The model under review builds one solid part; all positions refer to its coordinate system, in mm. A direction names the side the tool comes from. Coordinates: 2 decimals unless noted, no trailing zeros. Order: outer loops, then holes, each group sorted by start corner. A loop starts at its lowest first (then second) coordinate and runs counter-clockwise, first axis right, second up. Notation, with made-up numbers: M 78,89 L 124,89 A22 ccw 124,100 Z; hole C 74.25,-17.5 d11. An arc over 180 degrees is marked long. Answer in a Markdown table with one row per item.
from build123d import *

# Parameters (mm, degrees)
F0_W     = 66
F0_H     = 50
F1_DEPTH = 50
F2_W     = 24
F2_H     = 15
F3_DEPTH = 66
F6_DEPTH = 66
F7_W     = 16
F7_H     = 16
F8_DEPTH = 50


with BuildPart() as f1:
    # F0 (on Top) → F1 (new body)
    with BuildSketch(Plane.XY):
        with Locations((-18.661186, 12.861842)):
            Rectangle(F0_W, F0_H)
    extrude(amount=F1_DEPTH)

    # F2 (on face) → F3 (cut)
    with BuildSketch(Plane.YZ.offset(14.338814)):
        with Locations((12.148024, 42.5)):
            Rectangle(F2_W, F2_H)
    extrude(amount=-F3_DEPTH, mode=Mode.SUBTRACT)

    # F5 (on face) → F6 (cut)
    with BuildSketch(Plane.YZ.offset(14.338814)):
        with BuildLine():
            ThreePointArc((12.861842, 10.881519), (16.922608, 12.732394), (18.582238, 16.875001))
            ThreePointArc((18.582238, 16.875001), (8.241868, 21.017607), (12.861842, 10.881519))
        make_face()
    extrude(amount=-F6_DEPTH, mode=Mode.SUBTRACT)

    # F7 (on face) → F8 (cut)
    with BuildSketch(Plane.XY.offset(35)):
        with Locations((-33.807651, 12.345139)):
            Rectangle(F7_W, F7_H)
        with Locations((-3.504306, 12.252815)):
            Rectangle(F7_W, F7_H)
    extrude(amount=-F8_DEPTH, mode=Mode.SUBTRACT)


solid = f1.part
(1) Take a section at D-D (z = 27.5). Write out the cut boundary in (x, y).
Report:
| item | result |
|---|---|
| outline | M -51.66,-12.14 L 14.34,-12.14 L 14.34,37.86 L -51.66,37.86 Z; hole M -41.81,4.35 L -25.81,4.35 L -25.81,20.35 L -41.81,20.35 Z; hole M -11.5,4.25 L 4.5,4.25 L 4.5,20.25 L -11.5,20.25 Z |
(2) To check wall thickness, follow line 1 (X direction, y = 8, z = 7); line 2 (Y direction, x = -33, z = 31.5); line 3 (Y direction, x = -1.5, z = 37.5). State the ranges of each line that lie inside material, in increasing order. Write a range as [from, to].
Report:
| item | result |
|---|---|
| line 1 | [-51.66, -41.81], [-25.81, -11.5], [4.5, 14.34] |
| line 2 | [-12.14, 4.35], [20.35, 37.86] |
| line 3 | [-12.14, 0.15], [24.15, 37.86] |
(3) Take a section at A-A (x = -39). Write out the cut boundary in (y, z).
Report:
| item | result |
|---|---|
| outline | M -12.14,0 L 4.35,0 L 4.35,35 L 0.15,35 L 0.15,50 L -12.14,50 Z; M 20.35,0 L 37.86,0 L 37.86,50 L 24.15,50 L 24.15,35 L 20.35,35 Z |
(4) Take a section at C-C (y = 15). Write out the cut boundary in (x, z).
Report:
| item | result |
|---|---|
| outline | M -51.66,0 L -41.81,0 L -41.81,11.38 L -51.66,11.38 Z; M -51.66,22.37 L -41.81,22.37 L -41.81,35 L -51.66,35 Z; M -25.81,0 L -11.5,0 L -11.5,11.38 L -25.81,11.38 Z; M -25.81,22.37 L -11.5,22.37 L -11.5,35 L -25.81,35 Z; M 4.5,0 L 14.34,0 L 14.34,11.38 L 4.5,11.38 Z; M 4.5,22.37 L 14.34,22.37 L 14.34,35 L 4.5,35 Z |
(5) Machinability: for faces 4 (the flat face through (-18, 12, 35)), 5 (the flat face through (-19, 31, 50)), 6 (the flat face through (-41.808, 9, 22)), which of the approach directions +Z, -Z, +X, -X, +Y, -Y give a long, thin tool a straight path to every point of the face, cutting with its end or side? Answer none if there is none.
Report:
| item | result |
|---|---|
| face 4 | +Z, +X, -X |
| face 5 | +Z, +X, -X, +Y, -Y |
| face 6 | +Z, -Z |
(6) Insertion check: P1, Ø12, axis at x = -17.5, y = 8, coming from the +Z side. The pin has a flat end and moves straight along its axis. Give the tip position at first contact, or say it passes through.
Report:
| item | result |
|---|---|
| P1 | z = 35 |
(7) Take a section at B-B (z = 41). Write out the cut boundary in (x, y), then the cut area to 3 significant figures.
Report:
| item | result |
|---|---|
| outline | M -51.66,-12.14 L 14.34,-12.14 L 14.34,0.15 L -51.66,0.15 Z; M -51.66,24.15 L 14.34,24.15 L 14.34,37.86 L -51.66,37.86 Z |
| area | 1,720 mm^2 |
(8) The part is to be moulded in two halves that separate along X. For faces 1 (the flat face through (-51.661, 13, 25)), 2 (the flat face through (-19, -6, 50)), 3 (the flat face through (4.496, 9, 22)), say which applies: +X half, -X half, draft (parallel to the pull), parting line (faces both ways), or undercut.
Report:
| item | result |
|---|---|
| face 1 | -X half |
| face 2 | draft |
| face 3 | undercut |
